Check sheet for the modelled part. Datum: model origin and axes. Units: mm. A direction names the side the tool comes from. Round coordinates to 2 decimals unless told otherwise and drop trailing zeros. Order: outer loops, then holes, each group sorted by start corner. A loop starts at its lowest first (then second) coordinate and runs counter-clockwise, first axis right, second up.
```python
from build123d import *

# Parameters (mm, degrees)
F0_W     = 112.482
F0_H     = 130.175
F0_R     = 1.727
F0_R_2   = 36.003
F1_DEPTH = 33.25
F2_R     = 5
F3_DEPTH = 20
F4_R     = 5
F5_DEPTH = 20
F6_R     = 42.045
F7_DEPTH = 1.53


with BuildPart() as f1:
    # F0 (on Front) → F1 (new body)
    with BuildSketch(Plane.XZ):
        Rectangle(F0_W, F0_H)
        with Locations((-38.800708, -25.5)):
            Circle(F0_R, mode=Mode.SUBTRACT)
        with Locations((25.5, -38.800708)):
            Circle(F0_R, mode=Mode.SUBTRACT)
        with Locations((-25.5, 38.800708)):
            Circle(F0_R, mode=Mode.SUBTRACT)
        with Locations((0, 0)):
            Circle(F0_R_2, mode=Mode.SUBTRACT)
        with Locations((38.800708, 25.5)):
            Circle(F0_R, mode=Mode.SUBTRACT)
    extrude(amount=F1_DEPTH)

    # F2 (on face) → F3 (cut)
    with BuildSketch(Plane(origin=(-56.241, 0, 0), x_dir=(0, -1, 0), z_dir=(-1, 0, 0))):
        with Locations((16.625, 42.0525)):
            Circle(F2_R)
        with Locations((16.625, 14.0175)):
            Circle(F2_R)
        with Locations((16.625, -14.0175)):
            Circle(F2_R)
        with Locations((16.625, -42.0525)):
            Circle(F2_R)
    extrude(amount=-F3_DEPTH, mode=Mode.SUBTRACT)

    # F4 (on face) → F5 (cut)
    with BuildSketch(Plane.YZ.offset(56.241)):
        with Locations((-16.625, 42.0525)):
            Circle(F4_R)
        with Locations((-16.625, 14.0175)):
            Circle(F4_R)
        with Locations((-16.625, -14.0175)):
            Circle(F4_R)
        with Locations((-16.625, -42.0525)):
            Circle(F4_R)
    extrude(amount=-F5_DEPTH, mode=Mode.SUBTRACT)

    # F6 (on face) → F7 (cut)
    with BuildSketch(Plane(origin=(0, 0, 0), x_dir=(-1, 0, 0), z_dir=(0, 1, 0))):
        Circle(F6_R)
    extrude(amount=-F7_DEPTH, mode=Mode.SUBTRACT)


solid = f1.part
```
Item 1: Sectioned sample at C-C (z = -25.5). Record the cut outline in (x, y), and give its area (3 significant figures).
Answer:
outline: (-56.24, -33.25) - (-40.53, -33.25) - (-40.53, 0) - (-56.24, 0) - close; (-37.07, -33.25) - (-25.42, -33.25) - (-25.42, -1.53) - (-33.43, -1.53) - (-33.43, 0) - (-37.07, 0) - close; (25.42, -33.25) - (56.24, -33.25) - (56.24, 0) - (33.43, 0) - (33.43, -1.53) - (25.42, -1.53) - close
area: 1,910 mm2
Item 2: Release check for a two-part mould opening along X. For faces 1 (the flat face through (36.241, -17, -14)), 2 (the flat face through (-56.241, -16, -1)), 3 (the flat face through (-31, -1.53, 19)) record: released by +X, released by -X, zero draft, split by the parting line, or undercut.
Answer:
face 1: released by +X
face 2: released by -X
face 3: undercut
Item 3: Sectioned sample at D-D (x = 25.5). Record the cut outline in (y, z).
Answer:
outline: (-33.25, -65.09) - (0, -65.09) - (0, -40.53) - (-33.25, -40.53) - close; (-33.25, -37.07) - (0, -37.07) - (0, -33.43) - (-1.53, -33.43) - (-1.53, -25.42) - (-33.25, -25.42) - close; (-33.25, 25.42) - (-1.53, 25.42) - (-1.53, 33.43) - (0, 33.43) - (0, 65.09) - (-33.25, 65.09) - close
Item 4: Scan lines: line 1 along Z through (x, y) = (0, -19); line 2 along Z through (x, y) = (-24, -20); line 3 along X through (y, z) = (-12.5, 26.5). Record each from-to range of solid material in increasing order.
Answer:
line 1: z = -65.09 to -36, 36 to 65.09
line 2: z = -65.09 to -26.84, 26.84 to 37.94, 39.66 to 65.09
line 3: x = -56.24 to -24.37, 24.37 to 37.39, 40.21 to 56.24
Item 5: Go/stop test with flat-tipped pins: P1, Ø3, axis at x = 25.5, z = -38.8, coming from the +Y side; P2, Ø6, axis at y = -16.62, z = 14.02, coming from the +X side. Record where each tip stops, or that it passes through.
Answer:
P1: passes through
P2: stops at x = 36.24
Item 6: Sectioned sample at B-B (z = 0). Record the cut outline in (x, y) (3 decimals).
Answer:
outline: (-56.241, -33.25) - (-36.003, -33.25) - (-36.003, -1.53) - (-42.045, -1.53) - (-42.045, 0) - (-56.241, 0) - close; (36.003, -33.25) - (56.241, -33.25) - (56.241, 0) - (42.045, 0) - (42.045, -1.53) - (36.003, -1.53) - close
Item 7: Access from +Z, -Z, +X, -X, +Y, -Y to the whole of each face (thin tool, end or side, straight path). Record for faces 4 (the cylindrical face through (-37.205, -16.392, -26.161)), 5 (the cylindrical face through (46.4, -17.3, -37.1)), 6 (the cylindrical face through (-46.381, -21.394, -12.516)).
Answer:
face 4: +Y, -Y
face 5: +X
face 6: -X
